Verification items for the finished model (mm, model axes). A direction names the side the tool comes from. Give positions to 0.01 mm unless a question says otherwise; leave off trailing zeros. Loops run counter-clockwise (first coordinate to the right, second up) from the corner with the lowest first, then second, coordinate; pieces in that order, holes last. Notation, with made-up numbers: (-28, 43) -> (-9, 43) arc R21 ccw to (-9, 60) -> close; hole circle Ø8 at (31, 61.5). An arc over 180 degrees is marked (long way). Use one line per item in the form item = value. Start each with the question number.
from build123d import *

# Parameters (mm, degrees)
F0_R      = 65.900375
F1_DEPTH  = 28.702
F2_R      = 11.305854
F3_DEPTH  = 6.858
F4_R      = 18.635384
F5_DEPTH  = 6.096
F6_R      = 14.542748
F7_DEPTH  = 10.668
F8_R      = 11.447627
F9_DEPTH  = 3.048
F10_R     = 18.815081
F11_DEPTH = 5.08


with BuildPart() as f1:
    # F0 (on Top) → F1 (new body)
    with BuildSketch(Plane.XY):
        Circle(F0_R)
    extrude(amount=-F1_DEPTH)

    # F2 (on Top) → F3 (join)
    with BuildSketch(Plane.XY):
        with Locations((-15.24, 38.25875)):
            Circle(F2_R)
    extrude(amount=F3_DEPTH)

    # F4 (on Top) → F5 (join)
    with BuildSketch(Plane.XY):
        with Locations((-34.924999, -3.33375)):
            Circle(F4_R)
    extrude(amount=F5_DEPTH)

    # F6 (on Top) → F7 (join)
    with BuildSketch(Plane.XY):
        with Locations((25.400002, 15.08125)):
            Circle(F6_R)
    extrude(amount=F7_DEPTH)

    # F8 (on Top) → F9 (join)
    with BuildSketch(Plane.XY):
        with Locations((25.717501, -27.78125)):
            Circle(F8_R)
    extrude(amount=F9_DEPTH)

    # F10 (on Top) → F11 (join)
    with BuildSketch(Plane.XY):
        with Locations((-10.230287, -42.295363)):
            Circle(F10_R)
    extrude(amount=F11_DEPTH)


solid = f1.part
Item 1: Sectioned sample at D-D, the plane x = 35. Enter the section's corners in (y, z), and give its area (3 significant figures).
Item 2: Gauge pin test, flat ends, axial feed: pin 1 Ø4 at (x, z) = (-33.5, -14.5) entering from -Y; pin 2 Ø4 at (x, y) = (-10.5, 50.5) entering from +Z; pin 3 Ø19 at (x, y) = (-4, -51.5) entering from +Z. Record the tip position at first contact, or that the pin passes through.
Item 3: Sectioned sample at C-C, the plane z = -4. Enter the section's corners in (x, y).
Item 4: Material ranges on line 1 (Z direction, x = 37, y = 50.5); line 2 (Z direction, x = 0, y = -50); line 3 (Y direction, x = 35, z = 2.5), recorded low to high.
Item 5: Tool access check on faces 4 (the cylindrical face through (-24.1, -29.58, 2.5)), 5 (the flat face through (25, 15, 10.668)), 6 (the flat face through (26, -28, 3.048)), 7 (the flat face through (-35, -3, 6.096)). Record the directions out of +Z, -Z, +X, -X, +Y, -Y that give a thin tool (end or side, any length) a straight path to the whole face; none if there is none.
Item 6: Draft check along X on faces 1 (the cylindrical face through (31, -37.937, 1.503)), 2 (the cylindrical face through (-14.286, -64.333, -14.15)), 3 (the flat face through (-10, -42, 5.08)). Enter one of: +X half, -X half, draft (parallel to the pull), parting line (faces both ways), or undercut.
Item 7: Sectioned sample at A-A, the plane y = 43.5. Enter the section's corners in (x, z).
Item 8: Sectioned sample at B-B, the plane x = 0. Enter the section's corners in (y, z), and give its area (3 significant figures).
Outcome:
q1.outline = (-55.84, -28.7) -> (55.84, -28.7) -> (55.84, 0) -> (26.01, 0) -> (26.01, 10.67) -> (4.16, 10.67) -> (4.16, 0) -> (-21.08, 0) -> (-21.08, 3.05) -> (-34.48, 3.05) -> (-34.48, 0) -> (-55.84, 0) -> close
q1.area = 3,480 mm^2
q2.pin_1 = -57.88
q2.pin_2 = 6.86
q2.pin_3 = 5.08
q3.outline = circle Ø131.8 at (0, 0)
q4.line_1 = -28.7 to 0
q4.line_2 = -28.7 to 5.08
q4.line_3 = -34.48 to -21.08, 4.16 to 26.01
q5.face_4 = +Z
q5.face_5 = +Z, +X, -X, +Y, -Y
q5.face_6 = +Z, +X, -Y
q5.face_7 = +Z, -X, -Y
q6.face_1 = undercut
q6.face_2 = parting line
q6.face_3 = draft
q7.outline = (-49.5, -28.7) -> (49.5, -28.7) -> (49.5, 0) -> (-5.22, 0) -> (-5.22, 6.86) -> (-25.26, 6.86) -> (-25.26, 0) -> (-49.5, 0) -> close
q8.outline = (-65.9, -28.7) -> (65.9, -28.7) -> (65.9, 0) -> (-26.5, 0) -> (-26.5, 5.08) -> (-58.09, 5.08) -> (-58.09, 0) -> (-65.9, 0) -> close
q8.area = 3,940 mm^2
